Can you work these out from the model? Positions are in its coordinate system, mm. Face numbers are marked on the shaded views. A direction names the side the tool comes from. Give positions to 0.01 mm unless a question says otherwise; leave off trailing zeros. Loops run counter-clockwise (first coordinate to the right, second up) from the corner with the lowest first, then second, coordinate; pieces in that order, holes last. Notation, with made-up numbers: (8.5, 32) - (16.5, 32) arc R16 cw to (16.5, 59) - close; hole circle Ø2 at (51.25, 72). An arc over 180 degrees is marked (long way). Use a Markdown table: item, result. Add a question column.
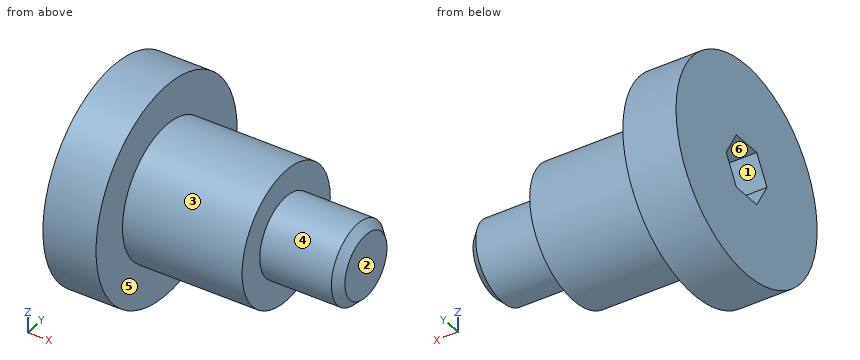
Autodesk Inventor part; units mm, degrees
ref_plane "YZ Plane" through (0, 0, 0) normal (1, 0, 0) x (0, 1, 0)
ref_plane "XZ Plane" through (0, 0, 0) normal (0, 1, 0) x (-1, 0, 0)
ref_plane "XY Plane" through (0, 0, 0) normal (0, 0, 1) x (1, 0, 0)
sketch "Sketch_1" plane through (0, 0, 0) normal (0, 0, 1) x (1, 0, 0)
  line L0 (4.5, 0) -> (-2, 0)
  line L1 (-2, 0) -> (-2, 4)
  line L2 (-2, 4) -> (0, 4)
  line L3 (0, 4) -> (0, 2.5)
  line L4 (0, 2.5) -> (4.5, 2.5)
  line L5 (4.5, 2.5) -> (4.5, 0)
  line L6 (4.5, 0) -> (-2, 0)
revolve "Revolution1" add sketch "Sketch_1" angle 360 about axis through (4.5, 0, 0) along (1, 0, 0)
sketch "Sketch2" plane through (-2, 0, 0) normal (-1, 0, 0) x (0, 0, 1)
  point P0 (0, 0)
hole "Hole1" at (-2, 0, 0) direction (1, 0, 0) diameter 2 depth 2 tip angle 120
sketch "Sketch_3" plane through (-2, 0, 0) normal (1, 0, 0) x (0, 0, -1)
  line L0 (-1, -0.5774) -> (0, -1.1547)
  line L1 (0, -1.1547) -> (1, -0.5774)
  line L2 (1, -0.5774) -> (1, 0.5774)
  line L3 (1, 0.5774) -> (0, 1.1547)
  line L4 (0, 1.1547) -> (-1, 0.5774)
  line L5 (-1, 0.5774) -> (-1, -0.5774)
extrude "Extrusion1" cut sketch "Sketch_3" along normal blind 2
sketch "Sketch_6" plane through (0, 0, 0) normal (0, 0, 1) x (1, 0, 0)
  line L0 (7.5, 0) -> (4.5, 0)
  line L1 (4.5, 0) -> (4.5, 1.5)
  line L2 (4.5, 1.5) -> (7.1935, 1.5)
  line L3 (7.1935, 1.5) -> (7.5, 1.1935)
  line L4 (7.5, 1.1935) -> (7.5, 0)
  line L5 (7.5, 0) -> (4.5, 0)
revolve "Revolution2" add sketch "Sketch_6" angle 360 about axis through (7.5, 0, 0) along (1, 0, 0)
thread "Thread1"
properties part number "DBTS3-4.5-3-LTC"
1. Will these pins go through, and if not, where does the flat tip stop? P1, Ø2, axis at x = 3, z = 1, coming from the -Y side; P2, Ø4, axis at x = 5, y = 2, coming from the -Z side; P3, Ø2, axis at x = 4.5, y = -0.5, coming from the +Z side.
2. Please list where these lines run through material, in increasing order: line 1 along X through (y, z) = (2, 2.5); line 2 along X through (y, z) = (-1.5, 0.5); line 3 along Z through (x, y) = (-0.25, 0.5). Write a range as [from, to].
3. Suppose I cut it at D-D (x = 6.5). List the corners of the cut face in (y, z) for me.
4. On a 3-axis mill with a long thin cutter (end or side, diameter ignored), from which of +Z, -Z, +X, -X, +Y, -Y can I reach the whole of each face in a straight line? I mean the marked faces 1, 2 and 3. Say none if no direction works.
5. Suppose I cut it at B-B (z = -2). List the corners of the cut face in (x, y) for me, and give its area (3 significant figures).
6. Suppose I cut it at C-C (y = -3). List the corners of the cut face in (x, z) for me, and give its area (3 significant figures).
7. Suppose I cut it at A-A (x = -1). List the corners of the cut face in (y, z) for me, and give its area (3 significant figures).
8. If we mould it in two halves opening along Z, with no side actions, what happens to the marked faces 4, 5 and 6? For each: released by +Z, released by -Z, zero draft, split by the parting line, or undercut.
Results below:
| question | item | result |
|---|---|---|
| 1 | P1 | y = -2.5 |
| 1 | P2 | z = -2.5 |
| 1 | P3 | z = 2.5 |
| 2 | line 1 | [-2, 0] |
| 2 | line 2 | [-2, 4.5] |
| 2 | line 3 | [-3.97, -1], [1, 3.97] |
| 3 | outline | circle Ø3 at (0, 0) |
| 4 | face 1 | -X |
| 4 | face 2 | +Z, -Z, +X, +Y, -Y |
| 4 | face 3 | +X |
| 5 | outline | (-2, -3.46) - (0, -3.46) - (0, -1.5) - (4.5, -1.5) - (4.5, 1.5) - (0, 1.5) - (0, 3.46) - (-2, 3.46) - close |
| 5 | area | 27.4 mm² |
| 6 | outline | (-2, -2.65) - (0, -2.65) - (0, 2.65) - (-2, 2.65) - close |
| 6 | area | 10.6 mm² |
| 7 | outline | circle Ø8 at (0, 0); hole (-1.15, 0) - (-0.58, -1) - (0.58, -1) - (1.15, 0) - (0.58, 1) - (-0.58, 1) - close |
| 7 | area | 46.8 mm² |
| 8 | face 4 | split by the parting line |
| 8 | face 5 | zero draft |
| 8 | face 6 | undercut |
